```python
from build123d import *

# Parameters (mm, degrees)
SKETCH1_R           = 37.5
BOSS_EXTRUDE1_DEPTH = 30
SKETCH2_R           = 25
BOSS_EXTRUDE2_DEPTH = 50
SKETCH3_R           = 10
BOSS_EXTRUDE3_DEPTH = 5
SKETCH4_R           = 50
BOSS_EXTRUDE4_DEPTH = 5
SKETCH5_R           = 2.5
CUT_EXTRUDE1_DEPTH  = 5


with BuildPart() as part:
    # Sketch1 → Boss-Extrude1 (new body)
    with BuildSketch(Plane(origin=(0, 0, 0), x_dir=(1, 0, 0), z_dir=(0, 1, 0))):
        with Locations(Location((0, 0, 0), (0, 0, 270))):
            Circle(SKETCH1_R)
    extrude(amount=BOSS_EXTRUDE1_DEPTH)

    # Sketch2 → Boss-Extrude2 (add)
    with BuildSketch(Plane(origin=(0, 30, 0), x_dir=(1, 0, 0), z_dir=(0, 1, 0))):
        with Locations(Location((0, 0, 0), (0, 0, 270))):
            Circle(SKETCH2_R)
    extrude(amount=BOSS_EXTRUDE2_DEPTH)

    # Sketch3 → Boss-Extrude3 (add)
    with BuildSketch(Plane(origin=(0, 80, 0), x_dir=(1, 0, 0), z_dir=(0, 1, 0))):
        with Locations(Location((0, 0, 0), (0, 0, 270))):
            Circle(SKETCH3_R)
    extrude(amount=BOSS_EXTRUDE3_DEPTH)

    # Sketch4 → Boss-Extrude4 (add)
    with BuildSketch(Plane.XZ):
        with Locations(Location((0, 0, 0), (0, 0, 270))):
            Circle(SKETCH4_R)
    extrude(amount=BOSS_EXTRUDE4_DEPTH)

    # Sketch5 → Cut-Extrude1 (cut)
    with BuildSketch(Plane.XZ.offset(5)):
        with Locations(Location((0, 45, 0), (0, 0, 270))):
            Circle(SKETCH5_R)
        with Locations(Location((38.97114317, 22.5, 0), (0, 0, 270))):
            Circle(SKETCH5_R)
        with Locations(Location((38.97114317, -22.5, 0), (0, 0, 270))):
            Circle(SKETCH5_R)
        with Locations(Location((0, -45, 0), (0, 0, 270))):
            Circle(SKETCH5_R)
        with Locations(Location((-38.97114317, -22.5, 0), (0, 0, 270))):
            Circle(SKETCH5_R)
        with Locations(Location((-38.97114317, 22.5, 0), (0, 0, 270))):
            Circle(SKETCH5_R)
    extrude(amount=-CUT_EXTRUDE1_DEPTH, mode=Mode.SUBTRACT)


solid = part.part
```
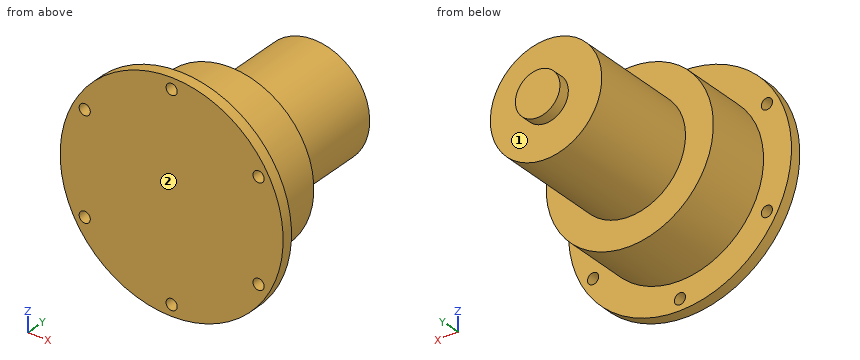
The model under review builds one solid part; all positions refer to its coordinate system, in mm. Face numbers are marked on the shaded views. A direction names the side the tool comes from. Round coordinates to 2 decimals unless told otherwise and drop trailing zeros. Loops run counter-clockwise (first coordinate to the right, second up) from the corner with the lowest first, then second, coordinate; pieces in that order, holes last. Notation, with made-up numbers: (25, 1) - (30, 1) arc R13 ccw to (30, 16) - close; hole circle Ø10 at (24, 31.5). An arc over 180 degrees is marked (long way). Use a Markdown table: item, result. Add a question column.
Q1. For probe 1 along X at (y, z) = (-1.9, -22.5); probe 2 along X at (y, z) = (-1, 22); probe 3 along Y at (x, z) = (36.5, 8), list the stretches that pass through material, from the lowest coordinate up.
Q2. Machinability: for the marked faces 1 and 2, which of the approach directions +Z, -Z, +X, -X, +Y, -Y give a long, thin tool a straight path to every point of the face, cutting with its end or side? Answer none if there is none.
Q3. Add section A-A (x = 0). State the section outline as (y, z) points.
Q4. Add section C-C (z = 0). State the section outline as (x, y) points, plus the area to 3 significant figures.
Q5. Add section B-B (z = 22.5). State the section outline as (x, y) points, plus the area to 3 significant figures.
Q6. Insertion check: pin 1 Ø8 at (y, z) = (14, 2.5) entering from -X; pin 2 Ø4 at (x, z) = (0, 45) entering from -Y; pin 3 Ø4 at (y, z) = (35, -2) entering from -X; pin 4 Ø12 at (y, z) = (57.5, -16) entering from +X. Each pin has a flat end and moves straight along its axis. Give the tip position at first contact, or say it passes through.
Q7. Add section D-D (y = 76). State the section outline as (x, z) points.
Worked answers:
| question | item | result |
|---|---|---|
| 1 | probe 1 | -44.65 to -41.47, -36.47 to 36.47, 41.47 to 44.65 |
| 1 | probe 2 | -44.9 to -41.42, -36.52 to 36.52, 41.42 to 44.9 |
| 1 | probe 3 | -5 to 30 |
| 2 | face 1 | +Y |
| 2 | face 2 | +Z, -Z, +X, -X, -Y |
| 3 | outline | (-5, -50) - (0, -50) - (0, -47.5) - (-5, -47.5) - close; (-5, -42.5) - (0, -42.5) - (0, -37.5) - (30, -37.5) - (30, -25) - (80, -25) - (80, -10) - (85, -10) - (85, 10) - (80, 10) - (80, 25) - (30, 25) - (30, 37.5) - (0, 37.5) - (0, 42.5) - (-5, 42.5) - close; (-5, 47.5) - (0, 47.5) - (0, 50) - (-5, 50) - close |
| 4 | outline | (-50, -5) - (50, -5) - (50, 0) - (37.5, 0) - (37.5, 30) - (25, 30) - (25, 80) - (10, 80) - (10, 85) - (-10, 85) - (-10, 80) - (-25, 80) - (-25, 30) - (-37.5, 30) - (-37.5, 0) - (-50, 0) - close |
| 4 | area | 5,350 mm² |
| 5 | outline | (-44.65, -5) - (-41.47, -5) - (-41.47, 0) - (-44.65, 0) - close; (-36.47, -5) - (36.47, -5) - (36.47, 0) - (30, 0) - (30, 30) - (10.9, 30) - (10.9, 80) - (-10.9, 80) - (-10.9, 30) - (-30, 30) - (-30, 0) - (-36.47, 0) - close; (41.47, -5) - (44.65, -5) - (44.65, 0) - (41.47, 0) - close |
| 5 | area | 3,290 mm² |
| 6 | pin 1 | x = -37.5 |
| 6 | pin 2 | through |
| 6 | pin 3 | x = -25 |
| 6 | pin 4 | x = 22.91 |
| 7 | outline | circle Ø50 at (0, 0) |
